```python
from build123d import *

# Parameters (mm, degrees)
F0_W      = 52.766081
F0_H      = 46.285272
F1_DEPTH  = 25.4
F2_R      = 16.792402
F2_R_2    = 10.881349
F3_DEPTH  = 12.7
F3_FACE_R = 10.881349
F4_DEPTH  = 25.4
F5_W      = 4.748795
F5_H      = 46.285272
F6_DEPTH  = 25.4


with BuildPart() as f1:
    # F0 (on Front) → F1 (new body)
    with BuildSketch(Plane.XZ):
        with Locations((-26.38304, 23.142636)):
            Rectangle(F0_W, F0_H)
    extrude(amount=F1_DEPTH)

    # F2 (on face) → F3 (join)
    with BuildSketch(Plane.XZ.offset(25.4)):
        with Locations((-28.835148, 23.680672)):
            Circle(F2_R)
        with Locations((-28.835148, 23.680672)):
            Circle(F2_R_2, mode=Mode.SUBTRACT)
    extrude(amount=F3_DEPTH)

    # F3_face (on face) → F4 (cut)
    with BuildSketch(Plane(origin=(-28.835148, -25.4, 23.680672), x_dir=(1, 0, 0), z_dir=(0, -1, 0))):
        Circle(F3_FACE_R)
    extrude(amount=-F4_DEPTH, mode=Mode.SUBTRACT)

    # F5 (on face) → F6 (cut)
    with BuildSketch(Plane.XZ.offset(25.4)):
        with Locations((-2.374397, 23.142636)):
            Rectangle(F5_W, F5_H)
    extrude(amount=-F6_DEPTH, mode=Mode.SUBTRACT)


solid = f1.part
```
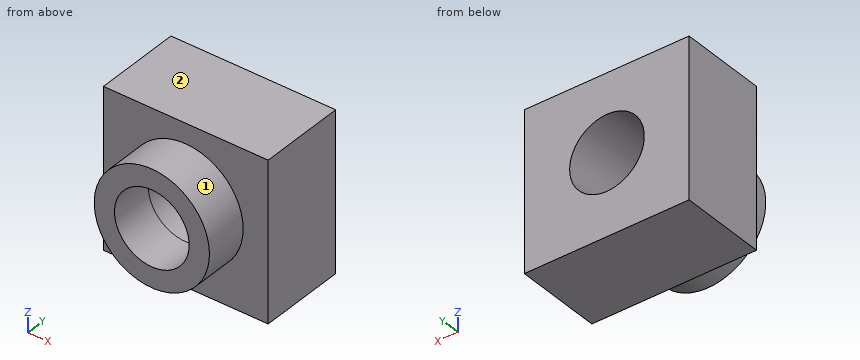
Model file for the job. Use its own axes, mm. Face numbers are marked on the shaded views. A direction names the side the tool comes from. Round coordinates to 2 decimals unless told otherwise and drop trailing zeros. Write each loop counter-clockwise with the first axis right and the second up, starting at its lowest first coordinate (ties: lowest second). Pieces come first, ordered by that corner, then holes. Notation, with made-up numbers: M 0,58 L 4,58 A35 cw 4,91 Z; hole C 52.5,55 d4. An arc over 180 degrees is marked long. Put each result on its own line as item: value.
Item 1: Cut at B-B (z = 15.5). List the corners of the cut face in (x, y).
Responses:
outline: M -52.77,-25.4 L -43.5,-25.4 L -43.5,-38.1 L -36.01,-38.1 L -36.01,0 L -52.77,0 Z; M -21.66,-38.1 L -14.17,-38.1 L -14.17,-25.4 L -4.75,-25.4 L -4.75,0 L -21.66,0 Z
Item 2: Cut at C-C (y = -9). List the corners of the cut face in (x, z).
Responses:
outline: M -52.77,0 L -4.75,0 L -4.75,46.29 L -52.77,46.29 Z; hole C -28.84,23.68 d21.76
Item 3: Flat gauge pins, fed straight in: P1, Ø1, axis at x = -12, z = 36, coming from the -Y side; P2, Ø5, axis at x = -15, y = -29, coming from the +Z side. Where does each tip first touch, or does it go through?
Responses:
P1: y = -25.4
P2: z = 36.07
Item 4: Cut at A-A (x = -28.5). List the corners of the cut face in (y, z).
Responses:
outline: M -38.1,6.89 L -25.4,6.89 L -25.4,0 L 0,0 L 0,12.8 L -38.1,12.8 Z; M -38.1,34.56 L 0,34.56 L 0,46.29 L -25.4,46.29 L -25.4,40.47 L -38.1,40.47 Z
Item 5: Tool access for the marked faces 1 and 2: list every direction of +Z, -Z, +X, -X, +Y, -Y with a clear straight run to the whole face (end or side of a thin tool).
Responses:
face 1: -Y
face 2: +Z, +X, -X, +Y, -Y
Item 6: Cut at D-D (x = -44). List the corners of the cut face in (y, z).
Responses:
outline: M -38.1,16.47 L -25.4,16.47 L -25.4,0 L 0,0 L 0,46.29 L -25.4,46.29 L -25.4,30.89 L -38.1,30.89 Z
Item 7: Probe L1, parallel to Y at x = -23, z = 5.5; L2, parallel to Z at x = -26, y = -24.5; L3, parallel to Z at x = -28.5, y = -12. List the from-to ranges inside material, lowest first. Write a range as from..to.
Responses:
L1: -25.4..0
L2: 0..13.18, 34.19..46.29
L3: 0..12.8, 34.56..46.29
